Build history of the part. All positions in model axes, mm. A direction names the side the tool comes from. Give positions to 0.01 mm unless a question says otherwise; leave off trailing zeros. Order: outer loops, then holes, each group sorted by start corner. A loop starts at its lowest first (then second) coordinate and runs counter-clockwise, first axis right, second up. Notation, with made-up numbers: (24, 34.5) - (31, 34.5) arc R20 ccw to (31, 55.5) - close; hole circle Ø11 at (-1, 7). An arc over 180 degrees is marked (long way). Use a Markdown table: item, result. Add a question column.
(1) Which spindle directions (+Z, -Z, +X, -X, +Y, -Y) get a long thin tool onto all of the face, cutting with end or side? Do faces 5 (the face through (20.99, 1.49, 11.52)), 6 (the face through (20.3, 0, -13.1)), 7 (the face through (-27.62, -5.15, 7.48)). Say none if no direction does.
(2) Slice it at A-A (x = 13.5). Write the cut outline in (y, z).
(3) Mould opens along X. For faces 1 (the face through (4, -3, 26.447)), 2 (the face through (37.378, 0.986, -13.567)), 3 (the face through (-29.608, -1, 8)), 4 (the face through (12, -6, 27)) say: +X half, -X half, draft (parallel to the pull), parting line (faces both ways), or undercut.
(4) Slice it at C-C (y = -0.75). Write the cut outline in (x, z), then the cut area to 3 significant figures.
(5) Flat gauge pins, fed straight in: pin 1 (8 mm diameter, centred on x = -5.5, z = 14.5, fed in from -Y); pin 2 (1.5 mm diameter, centred on y = -5, z = -13.5, fed in from +X). Where does each tip first touch, or does it go through?
(6) Wall check: line 1 (X direction, y = -4.5, z = 16.5); line 2 (Z direction, x = -3, y = -0.5); line 3 (X direction, y = -4, z = 2). Give the ranges that are in metal, low to high.
from build123d import *

# Parameters (mm, degrees)
SKETCH1_W            = 68
SKETCH1_H            = 44
BOSS_EXTRUDE1_DEPTH  = 2
SKETCH2_R            = 2
CUT_EXTRUDE1_DEPTH   = 2
SKETCH3_W            = 12
SKETCH3_H            = 23
CUT_EXTRUDE2_DEPTH   = 2
SKETCH4_W            = 3
SKETCH4_H            = 23
BOSS_EXTRUDE2_DEPTH  = 2
SKETCH8_W            = 6
SKETCH8_H            = 12
CUT_EXTRUDE4_DEPTH   = 20
CHAMFER2_SIZE        = 1
CHAMFER4_SIZE        = 2
SKETCH9_W            = 62
SKETCH9_H            = 38
BOSS_EXTRUDE5_DEPTH  = 6
CHAMFER5_SIZE        = 2
SKETCH12_W           = 8.376373975
SKETCH12_H           = 18.223954528
BOSS_EXTRUDE10_DEPTH = 2
SKETCH15_W           = 3
SKETCH15_H           = 1.5
BOSS_EXTRUDE11_DEPTH = 12
CHAMFER7_SIZE        = 1
SKETCH16_W           = 9
SKETCH16_H           = 0.5
BOSS_EXTRUDE12_DEPTH = 11
SKETCH17_W           = 6
SKETCH17_H           = 6
CUT_EXTRUDE5_DEPTH   = 11
FILLET1_R            = 2
SKETCH18_W           = 11
SKETCH18_H           = 3
CUT_EXTRUDE6_DEPTH   = 1
CHAMFER8_SIZE        = 1
SKETCH19_R           = 3.25
CUT_EXTRUDE7_DEPTH   = 11
CUT_EXTRUDE8_DEPTH   = 11
CHAMFER9_SIZE        = 1


with BuildPart() as part:
    # Sketch1 → Boss-Extrude1 (new body)
    with BuildSketch(Plane(origin=(0, 0, 0), x_dir=(1, 0, 0), z_dir=(0, 1, 0))):
        with Locations((4.391941392, -7.446886447)):
            Rectangle(SKETCH1_W, SKETCH1_H)
    extrude(amount=BOSS_EXTRUDE1_DEPTH)

    # Sketch2 → Cut-Extrude1 (cut)
    with BuildSketch(Plane(origin=(0, 2, 0), x_dir=(1, 0, 0), z_dir=(0, 1, 0))):
        with Locations(Location((-22.108058608, 7.253113553, 0), (0, 0, 270))):
            Circle(SKETCH2_R)
        with Locations(Location((31.091941392, 7.253113553, 0), (0, 0, 270))):
            Circle(SKETCH2_R)
        with Locations(Location((31.091941392, -22.146886447, 0), (0, 0, 270))):
            Circle(SKETCH2_R)
        with Locations(Location((-22.108058608, -22.146886447, 0), (0, 0, 270))):
            Circle(SKETCH2_R)
    extrude(amount=-CUT_EXTRUDE1_DEPTH, mode=Mode.SUBTRACT)

    # Sketch3 → Cut-Extrude2 (cut)
    with BuildSketch(Plane(origin=(0, 2, 0), x_dir=(1, 0, 0), z_dir=(0, 1, 0))):
        with Locations((32.391941392, -7.446886447)):
            Rectangle(SKETCH3_W, SKETCH3_H)
    extrude(amount=-CUT_EXTRUDE2_DEPTH, mode=Mode.SUBTRACT)

    # Sketch4 → Boss-Extrude2 (add)
    with BuildSketch(Plane(origin=(0, 2, 0), x_dir=(1, 0, 0), z_dir=(0, 1, 0))):
        with Locations((36.891941392, -7.446886447)):
            Rectangle(SKETCH4_W, SKETCH4_H)
    extrude(amount=-BOSS_EXTRUDE2_DEPTH)

    # Sketch8 → Cut-Extrude4 (cut)
    with BuildSketch(Plane(origin=(0, 2, 0), x_dir=(1, 0, 0), z_dir=(0, 1, 0))):
        with Locations((-26.608058608, -7.446886447)):
            Rectangle(SKETCH8_W, SKETCH8_H)
    extrude(amount=-CUT_EXTRUDE4_DEPTH, mode=Mode.SUBTRACT)

    # Chamfer2
    chamfer2_edges = [part.edges().sort_by_distance(p)[0] for p in [
        (-29.608058608, 1, 13.446886447),
        (-29.608058608, 1, 1.446886447),
    ]]
    chamfer(chamfer2_edges, length=CHAMFER2_SIZE)

    # Chamfer4
    chamfer4_edges = [part.edges().sort_by_distance(p)[0] for p in [
        (-29.608058608, 1, -14.553113553),
        (38.391941392, 1, -14.553113553),
        (38.391941392, 1, 29.446886447),
        (-29.608058608, 1, 29.446886447),
    ]]
    chamfer(chamfer4_edges, length=CHAMFER4_SIZE)

    # Sketch9 → Boss-Extrude5 (add)
    with BuildSketch(Plane.XZ):
        Polygon((-29.608058608, -14.553113553), (38.391941392, -14.553113553), (38.391941392, -11.553113553), (38.391941392, 25.764285426), (38.391941392, 29.446886447), (-29.608058608, 29.446886447), (-29.608058608, 25.764285426), (-29.608058608, -11.553113553), align=None)
        with Locations((4.391941392, 7.446886447)):
            Rectangle(SKETCH9_W, SKETCH9_H, mode=Mode.SUBTRACT)
    extrude(amount=BOSS_EXTRUDE5_DEPTH)

    # Chamfer5
    chamfer5_edges = [part.edges().sort_by_distance(p)[0] for p in [
        (38.391941392, -3, 29.446886447),
        (-29.608058608, -3, 29.446886447),
        (-29.608058608, -3, -14.553113553),
        (38.391941392, -3, -14.553113553),
    ]]
    chamfer(chamfer5_edges, length=CHAMFER5_SIZE - 0.0001)  # a hair under: the kernel refuses the full size

    # Sketch12 → Boss-Extrude10 (add)
    with BuildSketch(Plane(origin=(0, 2, 0), x_dir=(1, 0, 0), z_dir=(0, 1, 0))):
        with Locations((-25.419871621, -7.493021435)):
            Rectangle(SKETCH12_W, SKETCH12_H)
    extrude(amount=-BOSS_EXTRUDE10_DEPTH)

    # Sketch15 → Boss-Extrude11 (add)
    with BuildSketch(Plane(origin=(26.391941392, 0, 0), x_dir=(0, 0, -1), z_dir=(1, 0, 0))):
        with Locations((-7.446886447, 1.25)):
            Rectangle(SKETCH15_W, SKETCH15_H)
    extrude(amount=BOSS_EXTRUDE11_DEPTH)

    # Chamfer7
    chamfer7_edges = [part.edges().sort_by_distance(p)[0] for p in [
        (30.891941392, 0.5, 8.946886447),
        (30.891941392, 0.5, 5.946886447),
    ]]
    chamfer(chamfer7_edges, length=CHAMFER7_SIZE)

    # Sketch16 → Boss-Extrude12 (add)
    with BuildSketch(Plane(origin=(0, 0, 5.946886447), x_dir=(-1, 0, 0), z_dir=(0, 0, -1))):
        with Locations((-30.891941392, 1.75)):
            Rectangle(SKETCH16_W, SKETCH16_H)
    extrude(amount=BOSS_EXTRUDE12_DEPTH)

    # Sketch17 → Cut-Extrude5 (cut)
    with BuildSketch(Plane(origin=(0, 2, 0), x_dir=(1, 0, 0), z_dir=(0, 1, 0))):
        with Locations((23.391941392, -13.946886447)):
            Rectangle(SKETCH17_W, SKETCH17_H)
    extrude(amount=-CUT_EXTRUDE5_DEPTH, mode=Mode.SUBTRACT)

    # Fillet1
    fillet1_edges = [part.edges().sort_by_distance(p)[0] for p in [
        (20.391941392, 1, 16.946886447),
        (20.391941392, 1, 10.946886447),
    ]]
    fillet(fillet1_edges, radius=FILLET1_R)

    # Sketch18 → Cut-Extrude6 (cut)
    with BuildSketch(Plane.ZY.offset(29.608058608)):
        with Locations((7.446886447, -4.5)):
            Rectangle(SKETCH18_W, SKETCH18_H)
    extrude(amount=-CUT_EXTRUDE6_DEPTH, mode=Mode.SUBTRACT)

    # Chamfer8
    chamfer8_edges = [part.edges().sort_by_distance(p)[0] for p in [
        (-29.608058608, -4.5, 12.946886447),
        (-29.608058608, -3, 7.446886447),
        (-29.608058608, -4.5, 1.946886447),
    ]]
    chamfer(chamfer8_edges, length=CHAMFER8_SIZE - 0.0001)  # a hair under: the kernel refuses the full size

    # Sketch19 → Cut-Extrude7 (cut)
    with BuildSketch(Plane.ZY.offset(28.608058608)):
        with Locations((7.446886447, -8.4)):
            Circle(SKETCH19_R)
    extrude(amount=-CUT_EXTRUDE7_DEPTH, mode=Mode.SUBTRACT)

    # Sketch20 → Cut-Extrude8 (cut)
    with BuildSketch(Plane(origin=(0, 0, -14.553113553), x_dir=(-1, 0, 0), z_dir=(0, 0, -1))):
        with BuildLine():
            Line((-23.141941392, -2.75), (-23.141941392, -6))
            Line((-23.141941392, -6), (-17.641941392, -6))
            Line((-17.641941392, -6), (-17.641941392, -2.75))
            ThreePointArc((-17.641941392, -2.75), (-20.391941392, 0), (-23.141941392, -2.75))
        make_face()
    extrude(amount=-CUT_EXTRUDE8_DEPTH, mode=Mode.SUBTRACT)

    # Chamfer9
    chamfer9_edges = [part.edges().sort_by_distance(p)[0] for p in [
        (24.391941392, 0, 10.946886447),
        (20.391941392, 0, 13.946886447),
        (24.391941392, 0, 16.946886447),
        (20.97772783, 0, 11.532672885),
        (20.97772783, 0, 16.361100009),
    ]]
    chamfer(chamfer9_edges, length=CHAMFER9_SIZE)


solid = part.part
Solution:
| question | item | result |
|---|---|---|
| 1 | face 5 | +Y, -Y |
| 1 | face 6 | -Z, -Y |
| 1 | face 7 | -X, -Y |
| 2 | outline | (-6, -14.55) - (2, -14.55) - (2, 29.45) - (-6, 29.45) - (-6, 26.45) - (0, 26.45) - (0, -11.55) - (-6, -11.55) - close |
| 3 | face 1 | undercut |
| 3 | face 2 | +X half |
| 3 | face 3 | -X half |
| 3 | face 4 | draft |
| 4 | outline | (-29.61, -12.55) - (-27.61, -14.55) - (18.5, -14.55) - (18.5, -11.55) - (-26.61, -11.55) - (-26.61, 26.45) - (35.39, 26.45) - (35.39, -11.55) - (22.28, -11.55) - (22.28, -14.55) - (36.39, -14.55) - (38.39, -12.55) - (38.39, 27.45) - (36.39, 29.45) - (-27.61, 29.45) - (-29.61, 27.45) - close |
| 4 | area | 617 mm2 |
| 5 | pin 1 | y = 0 |
| 5 | pin 2 | x = 38.2 |
| 6 | line 1 | -29.61 to -26.61, 35.39 to 38.39 |
| 6 | line 2 | -14.55 to -11.55, 26.45 to 29.45 |
| 6 | line 3 | -28.61 to -26.61, 35.39 to 38.39 |
